from build123d import *

# Parameters (mm, degrees)
SKETCH_1_W      = 4
SKETCH_1_H      = 20
EXTRUDE_1_DEPTH = 4


with BuildPart() as part:
    # Эскиз1 → Бобышка-Вытянуть1 (new body)
    # profile 1 of 4: a face of its own
    with BuildSketch(Plane.XY):
        with BuildLine():
            Line((-60, 45), (-22.360679775, 45))
            ThreePointArc((-22.360679775, 45), (-18.27819687, 44.128709292), (-14.90711985, 41.666666667))
            ThreePointArc((-14.90711985, 41.666666667), (0, 35), (14.90711985, 41.666666667))
            ThreePointArc((14.90711985, 41.666666667), (18.27819687, 44.128709292), (22.360679775, 45))
            Line((22.360679775, 45), (60, 45))
            Line((60, 45), (60, -45))
            Line((60, -45), (-60, -45))
            Line((-60, -45), (-60, 45))
        make_face()
        with BuildLine():
            ThreePointArc((0, 8.325008306), (-11.322126202, 15.697320009), (-21.693624825, 7.038593896))
            ThreePointArc((-21.693624825, 7.038593896), (-21.780397742, -0.950934053), (-17.546591805, -7.726992913))
            ThreePointArc((-17.546591805, -7.726992913), (-14.298596462, -10.729197825), (-11.163444206, -13.849058145))
            ThreePointArc((-11.163444206, -13.849058145), (-5.512041052, -19.820511257), (0, -25.920840209))
            ThreePointArc((0, -25.920840209), (5.512041052, -19.820511257), (11.163444206, -13.849058145))
            ThreePointArc((11.163444206, -13.849058145), (14.298596462, -10.729197825), (17.546591805, -7.726992913))
            ThreePointArc((17.546591805, -7.726992913), (21.780397742, -0.950934053), (21.693624825, 7.038593896))
            ThreePointArc((21.693624825, 7.038593896), (11.322126202, 15.697320009), (0, 8.325008306))
        make_face(mode=Mode.SUBTRACT)
    # profile 2 of 4: a face of its own
    with BuildSketch(Plane.XY):
        with Locations((-62, -25.5)):
            Rectangle(SKETCH_1_W, SKETCH_1_H)
    # profile 3 of 4: a face of its own
    with BuildSketch(Plane.XY):
        with Locations((-62, 25.5)):
            Rectangle(SKETCH_1_W, SKETCH_1_H)
    # profile 4 of 4: a face of its own
    with BuildSketch(Plane.XY):
        with Locations((62, -7)):
            Rectangle(SKETCH_1_W, SKETCH_1_H)
    extrude(amount=EXTRUDE_1_DEPTH)


solid = part.part
Build history of the part. All positions in model axes, mm. A direction names the side the tool comes from. Round coordinates to 2 decimals unless told otherwise and drop trailing zeros. Loops run counter-clockwise (first coordinate to the right, second up) from the corner with the lowest first, then second, coordinate; pieces in that order, holes last. Notation, with made-up numbers: (16.5, 54.5) -> (37.5, 54.5) arc R15 ccw to (37.5, 69.5) -> close; hole circle Ø4 at (-27.5, 14). An arc over 180 degrees is marked (long way). One line per item, written item: value. Start each with the question number.
Q1. Probe line 1 along X through (y, z) = (28, 3.2); line 2 along X through (y, z) = (13, 0.6); line 3 along X through (y, z) = (-6, 3.4). List the from-to ranges inside material, lowest first.
Q2. Cut at A-A on y = 39. List the corners of the cut face in (x, z).
Q3. Cut at C-C on z = 3.4. List the corners of the cut face in (x, y) (3 decimals), plus the area to 3 significant figures.
Q4. Two-plate mould, pull along Y, no slides. Class faces 6 (the face through (-5.59, -19.736, 1.972)), 7 (the face through (-60, 40, 2)), 8 (the face through (1, -45, 2)): released by +Y, released by -Y, zero draft, split by the parting line, or undercut.
Q5. Drop flat-ended pins along their axis: pin 1 Ø1.2 at (y, z) = (38, 2.5) entering from -X; pin 2 Ø2 at (x, z) = (-63, 1.5) entering from +Y; pin 3 Ø1.2 at (y, z) = (23.5, 2) entering from +X. Give the stop position or say it passes through.
Q6. Cut at D-D on y = -32. List the corners of the cut face in (x, z).
Q7. Cut at B-B on x = 6.5. List the corners of the cut face in (y, z).
Q8. 3-axis set-ups, long thin cutter, end or side, ignore diameter. For faces 1 (the face through (-62, 15.5, 2)), 2 (the face through (-18, 44, 2)), 3 (the face through (-62, 35.5, 2)), 4 (the face through (21.75, -1.06, 1.97)), 5 (the face through (-62, -35.5, 2)): which of +Z, -Z, +X, -X, +Y, -Y reach the whole face in a straight line?
Computed:
1. line 1: -64 to 60
1. line 2: -60 to -18.02, -3.27 to 3.27, 18.02 to 60
1. line 3: -60 to -19.19, 19.19 to 64
2. outline: (-60, 0) -> (-12, 0) -> (-12, 4) -> (-60, 4) -> close; (12, 0) -> (60, 0) -> (60, 4) -> (12, 4) -> close
3. outline: (-64, -35.5) -> (-60, -35.5) -> (-60, -45) -> (60, -45) -> (60, -17) -> (64, -17) -> (64, 3) -> (60, 3) -> (60, 45) -> (22.361, 45) arc R10 ccw to (14.907, 41.667) arc R20 cw to (-14.907, 41.667) arc R10 ccw to (-22.361, 45) -> (-60, 45) -> (-60, 35.5) -> (-64, 35.5) -> (-64, 15.5) -> (-60, 15.5) -> (-60, -15.5) -> (-64, -15.5) -> close; hole (-21.694, 7.039) arc R14.225 ccw to (-17.547, -7.727) arc R120 cw to (-11.163, -13.849) arc R356.113 cw to (0, -25.921) arc R356.113 cw to (11.163, -13.849) arc R120 cw to (17.547, -7.727) arc R14.225 ccw to (21.694, 7.039) arc R11.367 ccw to (0, 8.325) arc R11.367 ccw to start
3. area: 9,570 mm²
4. face 6: undercut
4. face 7: zero draft
4. face 8: released by -Y
5. pin 1: x = -60
5. pin 2: y = 35.5
5. pin 3: x = 60
6. outline: (-64, 0) -> (60, 0) -> (60, 4) -> (-64, 4) -> close
7. outline: (-45, 0) -> (-18.76, 0) -> (-18.76, 4) -> (-45, 4) -> close; (14.93, 0) -> (36.09, 0) -> (36.09, 4) -> (14.93, 4) -> close
8. face 1: +Z, -Z, -X
8. face 2: +Z, -Z, +Y
8. face 3: +Z, -Z, -X, +Y
8. face 4: +Z, -Z
8. face 5: +Z, -Z, -X, -Y
